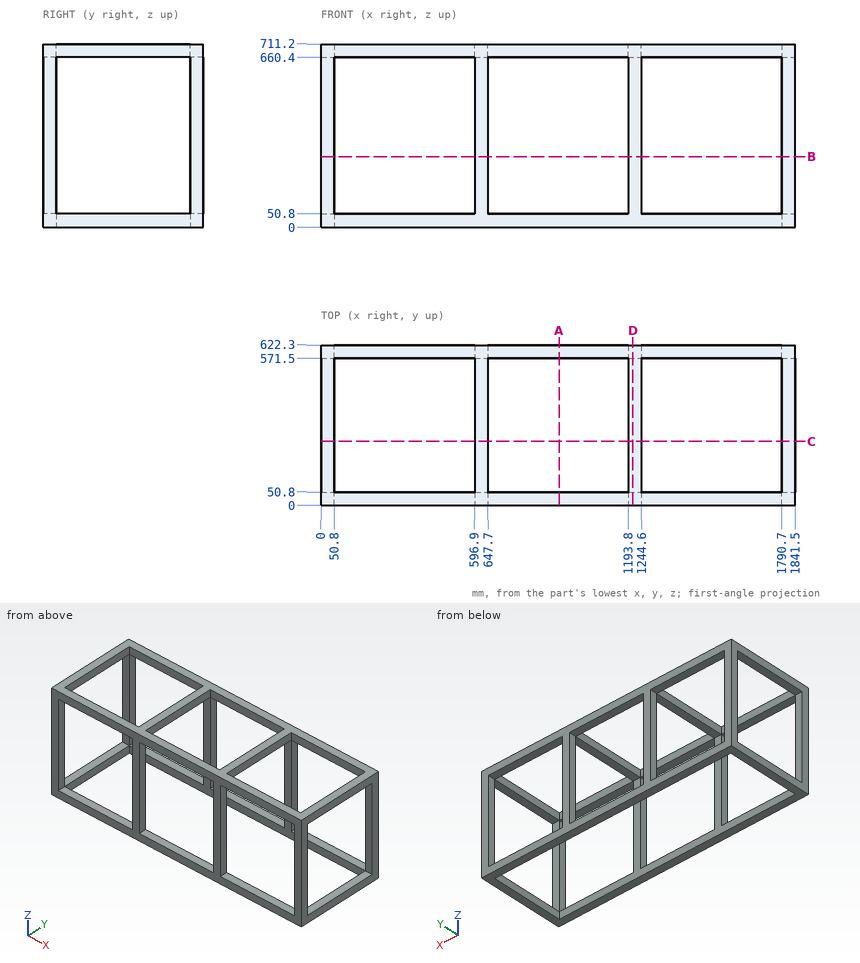
Job drawing, mm, ordinate dimensions from the low corner. One solid piece. Give positions to 0.01 mm unless a question says otherwise; leave off trailing zeros. Write each loop counter-clockwise with the first axis right and the second up, starting at its lowest first coordinate (ties: lowest second). Pieces come first, ordered by that corner, then holes. Notation, with made-up numbers: M 71.5,6.5 L 89.5,6.5 A35 cw 89.5,40.5 Z; hole C 84.5,-23.75 d11. An arc over 180 degrees is marked long. One line per item, written item: value. Start each with the question number.
Q1. Saw through at C-C, the plane y = 247.5. Write the cut outline in (x, z).
Q2. Saw through at A-A, the plane x = 924.5. Write the cut outline in (y, z), plus the area to 3 significant figures.
Q3. Saw through at D-D, the plane x = 1211. Write the cut outline in (y, z).
Q4. Saw through at B-B, the plane z = 273.5. State how many separate pieces and enclosed holes the cut face has, plus the area to 3 significant figures.
Q5. Probe probe 1 along X at (y, z) = (591, 264); probe 2 along Z at (x, y) = (1029, 25). List the from-to ranges inside material, lowest first. Write a range as [from, to].
Output values:
1. outline: M 0,0 L 50.8,0 L 50.8,50.8 L 0,50.8 Z; M 0,660.4 L 50.8,660.4 L 50.8,711.2 L 0,711.2 Z; M 596.9,660.4 L 647.7,660.4 L 647.7,711.2 L 596.9,711.2 Z; M 1193.8,660.4 L 1244.6,660.4 L 1244.6,711.2 L 1193.8,711.2 Z; M 1790.7,0 L 1841.5,0 L 1841.5,50.8 L 1790.7,50.8 Z; M 1790.7,660.4 L 1841.5,660.4 L 1841.5,711.2 L 1790.7,711.2 Z
2. outline: M 0,0 L 50.8,0 L 50.8,50.8 L 0,50.8 Z; M 0,660.4 L 50.8,660.4 L 50.8,711.2 L 0,711.2 Z; M 571.5,0 L 622.3,0 L 622.3,50.8 L 571.5,50.8 Z; M 571.5,660.4 L 622.3,660.4 L 622.3,711.2 L 571.5,711.2 Z
2. area: 10,300 mm²
3. outline: M 0,0 L 50.8,0 L 50.8,660.4 L 571.5,660.4 L 571.5,0 L 622.3,0 L 622.3,711.2 L 0,711.2 Z
4. separate pieces: 8
4. enclosed holes: 0
4. area: 20,600 mm²
5. probe 1: x = [0, 50.8], [596.9, 647.7], [1193.8, 1244.6], [1790.7, 1841.5]
5. probe 2: z = [0, 50.8], [660.4, 711.2]
